Source: CAD feature listing. Evaluate the final solid. Frame: model axes, mm. Coordinates: 2 decimals unless noted, no trailing zeros. Order: outer loops, then holes, each group sorted by start corner. A loop starts at its lowest first (then second) coordinate and runs counter-clockwise, first axis right, second up. Notation, with made-up numbers: (76.5, 28.5) - (123.5, 28.5) arc R21 cw to (123.5, 56.5) - close; hole circle Ø5 at (79, -34). An arc over 180 degrees is marked (long way). One line per question, with ' | ' between items. Start each with the question number.
(1) Section A-A (x = 287.5). Return the cut outline in (y, z), then the cut area to 3 significant figures.
(2) Line query: line 1 along Y through (x, z) = (424.5, 104.5); line 2 along X through (y, z) = (1.65, -2.5) (3 decimals); line 3 along Z through (x, y) = (343, 1.7). Output: solid intervals per line, ascending.
(3) Section C-C (y = 1.55). Return the cut outline in (x, z), then the cut area to 3 significant figures.
(4) Section D-D (x = 385.5). Return the cut outline in (y, z), then the cut area to 3 significant figures.
(5) Contact query for flat-ended pins moving along their axis: P1, Ø1.5, axis at y = 0.5, z = 53.5, coming from the -X side; P2, Ø14.5, axis at x = 347.27, z = -3.61, coming from the -Y side; P3, Ø10, axis at x = 424.5, z = 82, coming from the +Y side. Output: stop coordinate, or through.
(6) Section B-B (z = 12). Return the cut outline in (x, y).
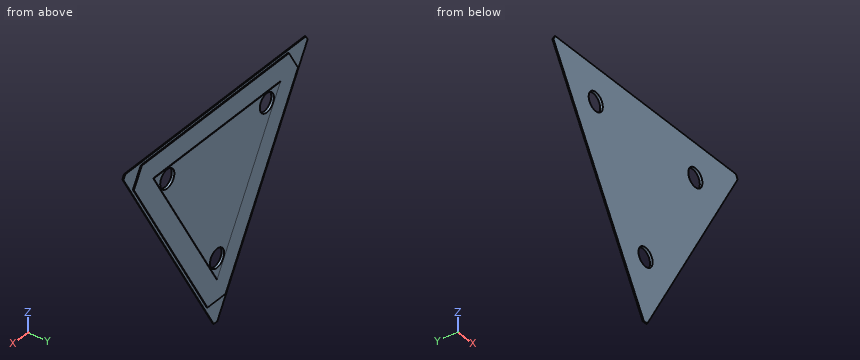
from build123d import *

# Parameters (mm, degrees)
BOSS_EXTRUDE1_DEPTH = 1
BOSS_EXTRUDE2_DEPTH = 2
SKETCH1_13_R        = 9
BOSS_EXTRUDE3_DEPTH = 2.5


with BuildPart() as part:
    # Sketch1 → Boss-Extrude1 (new body)
    with BuildSketch(Plane(origin=(0, 0, 0), x_dir=(1, 0, 0), z_dir=(0, 1, 0))):
        Polygon((464.784783451, -134.986661544), (462.517056767, -138.914415757), (231.981171214, -138.914415757), (229.712705007, -134.986323544), (344.980692969, 64.663360453), (349.516789508, 64.663360453), align=None)
        Polygon((452.699916625, -118.984688015), (442.602090749, -136.409305398), (254.809280576, -136.408896139), (243.304219773, -116.484791866), (335.767496284, 43.666038066), (358.778179035, 43.666038066), align=None, mode=Mode.SUBTRACT)
    extrude(amount=BOSS_EXTRUDE1_DEPTH)

    # Sketch1_12 → Boss-Extrude2 (add)
    with BuildSketch(Plane(origin=(0, 0, 0), x_dir=(1, 0, 0), z_dir=(0, 1, 0))):
        Polygon((442.602090749, -136.409305398), (254.809280576, -136.408896139), (243.304219773, -116.484791866), (335.767496284, 43.666038066), (358.778179035, 43.666038066), (452.699916625, -118.984688015), align=None)
        Polygon((266.439108268, -116.428009241), (428.113670918, -116.417164681), (347.273609729, 23.609230825), align=None, mode=Mode.SUBTRACT)
    extrude(amount=BOSS_EXTRUDE2_DEPTH)

    # Sketch1_13 → Boss-Extrude3 (add)
    with BuildSketch(Plane(origin=(0, 0, 0), x_dir=(1, 0, 0), z_dir=(0, 1, 0))):
        Polygon((266.439108268, -116.428009241), (428.113670918, -116.417164681), (347.273609729, 23.609230825), align=None)
        with Locations(Location((347.273609729, 3.609230825, 0), (0, 0, 270))):
            Circle(SKETCH1_13_R, mode=Mode.SUBTRACT)
        with Locations(Location((410.793152563, -106.417182487, 0), (0, 0, 270))):
            Circle(SKETCH1_13_R, mode=Mode.SUBTRACT)
        with Locations(Location((283.758521159, -106.426112565, 0), (0, 0, 270))):
            Circle(SKETCH1_13_R, mode=Mode.SUBTRACT)
    extrude(amount=BOSS_EXTRUDE3_DEPTH)


solid = part.part
Response values:
1) outline: (0, 34.9) - (1, 34.9) - (1, 39.94) - (2, 39.94) - (2, 79.94) - (2.5, 79.94) - (2.5, 98.24) - (0, 98.24) - close; (0, 114.61) - (2.5, 114.61) - (2.5, 116.43) - (2, 116.43) - (2, 136.41) - (1, 136.41) - (1, 138.91) - (0, 138.91) - close | area: 178 mm²
2) line 1: y = 0 to 2 | line 2: x = 312 to 338.342, 356.205 to 382.549 | line 3: z = -43.67 to -11.53, 4.31 to 136.41
3) outline: (243.3, 116.48) - (335.77, -43.67) - (358.78, -43.67) - (452.7, 118.98) - (442.6, 136.41) - (254.81, 136.41) - close; hole circle Ø18 at (283.76, 106.43); hole circle Ø18 at (347.27, -3.61); hole circle Ø18 at (410.79, 106.42) | area: 21,700 mm²
4) outline: (0, -2.34) - (1, -2.34) - (1, 2.61) - (2, 2.61) - (2, 42.6) - (2.5, 42.6) - (2.5, 116.42) - (2, 116.42) - (2, 136.41) - (1, 136.41) - (1, 138.91) - (0, 138.91) - close | area: 312 mm²
5) P1: stops at x = 276.33 | P2: passes through | P3: stops at y = 2
6) outline: (300.72, 0) - (393.78, 0) - (393.78, 1) - (390.92, 1) - (390.92, 2) - (367.83, 2) - (367.83, 2.5) - (326.72, 2.5) - (326.72, 2) - (303.63, 2) - (303.63, 1) - (300.72, 1) - close
